from build123d import *

# Parameters (mm, degrees)
BOSS_EXTRUDE1_DEPTH = 60
CUT_EXTRUDE1_DEPTH  = 10
SKETCH3_R           = 30
BOSS_EXTRUDE2_DEPTH = 30
SKETCH4_R           = 20
CUT_EXTRUDE3_DEPTH  = 20
SKETCH5_R           = 10
CUT_EXTRUDE4_DEPTH  = 129
SKETCH7_W           = 30
SKETCH7_H           = 5
BOSS_EXTRUDE3_DEPTH = 25
CUT_EXTRUDE5_DEPTH  = 20
SKETCH9_R           = 30
CUT_EXTRUDE6_DEPTH  = 10
SKETCH10_R          = 15
CUT_EXTRUDE7_DEPTH  = 155
CUT_EXTRUDE8_DEPTH  = 10


with BuildPart() as part:
    # Sketch1 → Boss-Extrude1 (new body)
    with BuildSketch(Plane.XY):
        with BuildLine():
            Line((0, 50), (100, 50))
            ThreePointArc((100, 50), (150, 0), (100, -50))
            Line((100, -50), (0, -50))
            ThreePointArc((0, -50), (-50, 0), (0, 50))
        make_face()
    extrude(amount=BOSS_EXTRUDE1_DEPTH)

    # Sketch2 → Cut-Extrude1 (cut)
    with BuildSketch(Plane(origin=(0, 0, 0), x_dir=(-1, 0, 0), z_dir=(0, 0, -1))):
        with BuildLine():
            Line((0, -30), (-100, -30))
            ThreePointArc((-100, -30), (-130, 0), (-100, 30))
            Line((-100, 30), (0, 30))
            ThreePointArc((0, 30), (30, 0), (0, -30))
        make_face()
    extrude(amount=-CUT_EXTRUDE1_DEPTH, mode=Mode.SUBTRACT)

    # Sketch3 → Boss-Extrude2 (add)
    with BuildSketch(Plane.XY.offset(60)):
        with Locations((100, 0)):
            Circle(SKETCH3_R)
    extrude(amount=BOSS_EXTRUDE2_DEPTH)

    # Sketch4 → Cut-Extrude3 (cut)
    with BuildSketch(Plane.XY.offset(90)):
        with Locations((100, 0)):
            Circle(SKETCH4_R)
    extrude(amount=-CUT_EXTRUDE3_DEPTH, mode=Mode.SUBTRACT)

    # Sketch5 → Cut-Extrude4 (cut)
    with BuildSketch(Plane.XY.offset(70)):
        with Locations((100, 0)):
            Circle(SKETCH5_R)
    extrude(amount=-CUT_EXTRUDE4_DEPTH, mode=Mode.SUBTRACT)

    # Sketch7 → Boss-Extrude3 (add)
    with BuildSketch(Plane.XY.offset(60)):
        with Locations((55.104348142, 0)):
            Rectangle(SKETCH7_W, SKETCH7_H)
    extrude(amount=BOSS_EXTRUDE3_DEPTH)

    # Sketch8 → Cut-Extrude5 (cut)
    with BuildSketch(Plane.XY.offset(60)):
        with BuildLine():
            ThreePointArc((-14, 48), (-40, 30), (-50, 0))
            Line((-50, 0), (-18, -24))
            ThreePointArc((-18, -24), (24, -18), (18, 24))
            Line((18, 24), (-14, 48))
        make_face()
    extrude(amount=-CUT_EXTRUDE5_DEPTH, mode=Mode.SUBTRACT)

    # Sketch9 → Cut-Extrude6 (cut)
    with BuildSketch(Plane.XY.offset(40)):
        Circle(SKETCH9_R)
    extrude(amount=-CUT_EXTRUDE6_DEPTH, mode=Mode.SUBTRACT)

    # Sketch10 → Cut-Extrude7 (cut)
    with BuildSketch(Plane.XY.offset(30)):
        Circle(SKETCH10_R)
    extrude(amount=-CUT_EXTRUDE7_DEPTH, mode=Mode.SUBTRACT)

    # Sketch11 → Cut-Extrude8 (cut)
    with BuildSketch(Plane.XZ.offset(2.5)):
        Polygon((40.104348142, 60), (70.104348142, 85), (40.104348142, 85), align=None)
    extrude(amount=-CUT_EXTRUDE8_DEPTH, mode=Mode.SUBTRACT)


solid = part.part
The model under review builds one solid part; all positions refer to its coordinate system, in mm. A direction names the side the tool comes from. Coordinates: 2 decimals unless noted, no trailing zeros. Write each loop counter-clockwise with the first axis right and the second up, starting at its lowest first coordinate (ties: lowest second). Pieces come first, ordered by that corner, then holes. Notation, with made-up numbers: M 62,-27.5 L 71,-27.5 A36 ccw 71,8.5 Z; hole C -34,-21 d10. An arc over 180 degrees is marked long. Put each result on its own line as item: value.
1) Add section B-B on z = 25. Give the boundary of the cut face in (x, y), then the cut area to 3 significant figures.
Computed:
outline: M 0,-50 L 100,-50 A50 ccw 100,50 L 0,50 A50 ccw Z; hole C 0,0 d30; hole C 100,0 d20
area: 16,800 mm2
2) Add section D-D on z = 66. Give the boundary of the cut face in (x, y).
Computed:
outline: M 47.3,-2.5 L 70.1,-2.5 A30 ccw long 70.1,2.5 L 47.3,2.5 Z; hole C 100,0 d20
3) Clearance check with flat-ended pins moving along their axes: pin 1 Ø12 at (x, y) = (92, -4) entering from +Z; pin 2 Ø8 at (x, z) = (58.5, 70) entering from +Y; pin 3 Ø10 at (y, z) = (11.5, 43.5) entering from +X; pin 4 Ø18 at (x, y) = (0, 0) entering from -Z. State where each tip first meets the part, or that it passes through.
Computed:
pin 1: stops at z = 70
pin 2: stops at y = 2.5
pin 3: stops at x = 149.58
pin 4: passes through
4) Wall thickness on probe 1 along Y at (x, z) = (100, 78.75); probe 2 along Y at (x, z) = (100, 49); probe 3 along Z at (x, y) = (89.5, 39): over which ranges is each line inside the solid? List them lowest first. Write a range as [from, to].
Computed:
probe 1: y = [-30, -20], [20, 30]
probe 2: y = [-50, -10], [10, 50]
probe 3: z = [0, 60]
5) Add section C-C on y = 37. Give the boundary of the cut face in (x, z), then the cut area to 3 significant figures.
Computed:
outline: M -33.63,0 L 133.63,0 L 133.63,60 L 0.67,60 L 0.67,40 L -33.63,40 Z
area: 9,350 mm2
6) Draft analysis for pull direction Y (two halves, no side actions). For faces 1 (the flat face through (62, 2.5, 67)), 2 (the cylindrical face through (129.993, -0.66, 4.93)), 3 (the cylindrical face through (149.988, 1.099, 29.58)), state which applies: released by +Y, released by -Y, zero draft, split by the parting line, or undercut.
Computed:
face 1: released by +Y
face 2: undercut
face 3: split by the parting line
7) Add section A-A on x = 106. Give the boundary of the cut face in (y, z).
Computed:
outline: M -49.64,0 L -29.39,0 L -29.39,10 L -8,10 L -8,70 L -19.08,70 L -19.08,90 L -29.39,90 L -29.39,60 L -49.64,60 Z; M 8,10 L 29.39,10 L 29.39,0 L 49.64,0 L 49.64,60 L 29.39,60 L 29.39,90 L 19.08,90 L 19.08,70 L 8,70 Z
8) For faces 4 (the flat face through (51, 30, 5)), 5 (the flat face through (-34, -12, 50)), 6 (the flat face through (6, 14, 30)), list the 3-axis set-ups (+Z, -Z, +X, -X, +Y, -Y) from which the entire face can be reached by the end or side of a thin tool; tool diameter is ignored.
Computed:
face 4: -Z
face 5: +Z, +Y
face 6: +Z
